Geometry: final body of the model. Coordinates: model frame, mm. Face numbers are marked on the shaded views. A direction names the side the tool comes from. Give positions to 0.01 mm unless a question says otherwise; leave off trailing zeros. Write each loop counter-clockwise with the first axis right and the second up, starting at its lowest first coordinate (ties: lowest second). Pieces come first, ordered by that corner, then holes.
from build123d import *

# Parameters (mm, degrees)
F1_DEPTH = 18


with BuildPart() as f1:
    # F0 (on Front) → F1 (new body)
    with BuildSketch(Plane.XZ):
        with BuildLine():
            ThreePointArc((-42.488194, 0), (-36.63033, 14.142136), (-22.488194, 20))
            Line((-22.488194, 20), (-2.488194, 20))
            Line((-2.488194, 20), (17.511806, 20))
            ThreePointArc((17.511806, 20), (31.653942, 14.142136), (37.511806, 0))
            Line((37.511806, 0), (42.511806, 0))
            ThreePointArc((42.511806, 0), (35.189476, 17.67767), (17.511806, 25))
            Line((17.511806, 25), (-2.488194, 25))
            Line((-2.488194, 25), (-22.488194, 25))
            ThreePointArc((-22.488194, 25), (-40.165863, 17.67767), (-47.488194, 0))
            Line((-47.488194, 0), (-42.488194, 0))
        make_face()
    extrude(amount=F1_DEPTH)


solid = f1.part
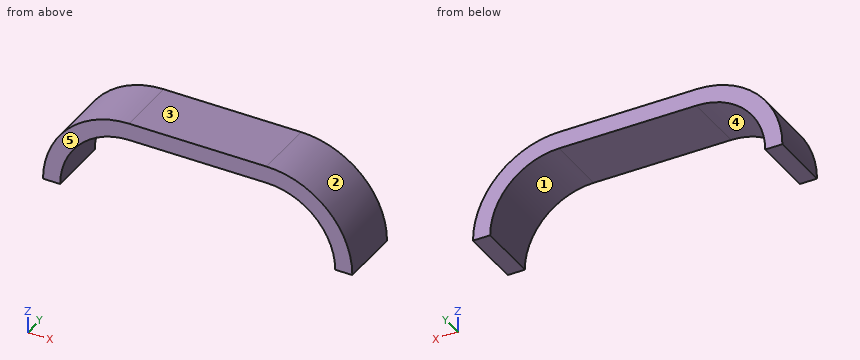
Q1. Access query for the marked faces 4 and 5. Directions: +Z, -Z, +X, -X, +Y, -Y. A direction counts if a zero-diameter tool reaches every point of the face in a straight line with its end or side. Return the directions, or none.
Filled sheet:
face 4: -Z, +Y, -Y
face 5: +Z, -Z, +X, -X, -Y
Q2. Section C-C on z = 16.75. Output: boundary loops of the cut face in (x, y).
Filled sheet:
outline: (-41.05, -18) - (-33.42, -18) - (-33.42, 0) - (-41.05, 0) - close; (28.44, -18) - (36.07, -18) - (36.07, 0) - (28.44, 0) - close
Q3. Section B-B on y = -9.5. Output: boundary loops of the cut face in (x, z).
Filled sheet:
outline: (-47.49, 0) - (-42.49, 0) arc R20 cw to (-22.49, 20) - (17.51, 20) arc R20 cw to (37.51, 0) - (42.51, 0) arc R25 ccw to (17.51, 25) - (-22.49, 25) arc R25 ccw to start
Q4. Section A-A on z = 4.25. Output: boundary loops of the cut face in (x, y).
Filled sheet:
outline: (-47.12, -18) - (-42.03, -18) - (-42.03, 0) - (-47.12, 0) - close; (37.06, -18) - (42.15, -18) - (42.15, 0) - (37.06, 0) - close
Q5. Section D-D on x = -4.5. Output: boundary loops of the cut face in (y, z).
Filled sheet:
outline: (-18, 20) - (0, 20) - (0, 25) - (-18, 25) - close
Q6. Pin query (flat end, axial travel): P1, Ø8, axis at x = -2, y = -12, coming from the -Z side; P2, Ø6, axis at y = -8, z = 13, coming from the +X side; P3, Ø6, axis at x = -37, y = -7, coming from the +Z side. Return the tip coordinate at first contact, or that it passes through.
Filled sheet:
P1: stops at z = 20
P2: stops at x = 40.42
P3: stops at z = 22.19
Q7. Pull-direction query (X, two-part tool) for the marked faces 1, 2 and 3; classes: released by +X, released by -X, zero draft, split by the parting line, or undercut.
Filled sheet:
face 1: undercut
face 2: released by +X
face 3: zero draft
Q8. Ray query, line 1 along X through (y, z) = (-16.75, 2.75); line 2 along X through (y, z) = (-3.75, 15.75); line 3 along Z through (x, y) = (7, -5). Return the intervals inside material, ascending.
Filled sheet:
line 1: x = -47.34 to -42.3, 37.32 to 42.36
line 2: x = -41.9 to -34.81, 29.84 to 36.93
line 3: z = 20 to 25
